from build123d import *

# Parameters (mm, degrees)
SKETCH2_W           = 18
SKETCH2_H           = 18
BOSS_EXTRUDE1_DEPTH = 18
SKETCH3_R           = 1.4224
CUT_EXTRUDE1_DEPTH  = 6.6
SKETCH4_R           = 1.4224
CUT_EXTRUDE2_DEPTH  = 6.6
SKETCH5_R           = 1.4224
CUT_EXTRUDE3_DEPTH  = 6.6
SKETCH6_W           = 16
SKETCH6_H           = 16
CUT_EXTRUDE4_DEPTH  = 16
SKETCH7_W           = 16
SKETCH7_H           = 16
CUT_EXTRUDE5_DEPTH  = 10


with BuildPart() as part:
    # Sketch2 → Boss-Extrude1 (new body)
    with BuildSketch(Plane(origin=(0, 0, 0), x_dir=(1, 0, 0), z_dir=(0, 1, 0))):
        Rectangle(SKETCH2_W, SKETCH2_H)
    extrude(amount=BOSS_EXTRUDE1_DEPTH)

    # Sketch3 → Cut-Extrude1 (cut)
    with BuildSketch(Plane(origin=(0, 18, 0), x_dir=(1, 0, 0), z_dir=(0, 1, 0))):
        Circle(SKETCH3_R)
    extrude(amount=-CUT_EXTRUDE1_DEPTH, mode=Mode.SUBTRACT)

    # Sketch4 → Cut-Extrude2 (cut)
    with BuildSketch(Plane(origin=(9, 0, 0), x_dir=(0, 0, -1), z_dir=(1, 0, 0))):
        with Locations((0, 9)):
            Circle(SKETCH4_R)
    extrude(amount=-CUT_EXTRUDE2_DEPTH, mode=Mode.SUBTRACT)

    # Sketch5 → Cut-Extrude3 (cut)
    with BuildSketch(Plane.XY.offset(9)):
        with Locations((0, 9)):
            Circle(SKETCH5_R)
    extrude(amount=-CUT_EXTRUDE3_DEPTH, mode=Mode.SUBTRACT)

    # Sketch6 → Cut-Extrude4 (cut)
    with BuildSketch(Plane(origin=(0, 0, -9), x_dir=(-1, 0, 0), z_dir=(0, 0, -1))):
        with Locations((1, 8)):
            Rectangle(SKETCH6_W, SKETCH6_H)
    extrude(amount=-CUT_EXTRUDE4_DEPTH, mode=Mode.SUBTRACT)

    # Sketch7 → Cut-Extrude5 (cut)
    with BuildSketch(Plane.ZY.offset(-7)):
        with Locations((-1, 8)):
            Rectangle(SKETCH7_W, SKETCH7_H)
    extrude(amount=-CUT_EXTRUDE5_DEPTH, mode=Mode.SUBTRACT)


solid = part.part
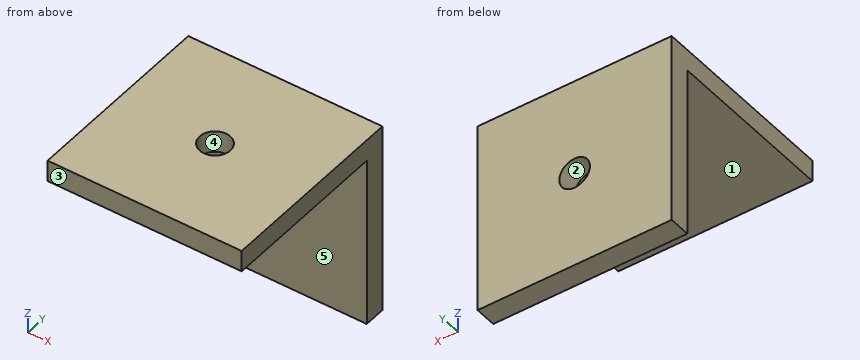
Model file for the job. Use its own axes, mm. Face numbers are marked on the shaded views. A direction names the side the tool comes from. Give positions to 0.01 mm unless a question says otherwise; leave off trailing zeros. Loops run counter-clockwise (first coordinate to the right, second up) from the corner with the lowest first, then second, coordinate; pieces in that order, holes last.
Item 1: Which spindle directions (+Z, -Z, +X, -X, +Y, -Y) get a long thin tool onto all of the face, cutting with end or side? Do the marked faces 4 and 5. Say none if no direction does.
Check values:
face 4: +Z, -Z
face 5: -Z, +X, -X, -Y
Item 2: Slice it at C-C (x = 0). Write the cut outline in (y, z).
Check values:
outline: (0, 7) - (7.58, 7) - (7.58, 9) - (0, 9) - close; (10.42, 7) - (16, 7) - (16, 1.42) - (18, 1.42) - (18, 9) - (10.42, 9) - close; (16, -9) - (18, -9) - (18, -1.42) - (16, -1.42) - close
Item 3: Drop flat-ended pins along their axis: P1, Ø5, axis at x = -2.5, y = 9, coming from the -Z side; P2, Ø2, axis at x = 4, z = 0.5, coming from the -Y side. Give the stop position or say it passes through.
Check values:
P1: stops at z = 7
P2: stops at y = 16
Item 4: Slice it at D-D (x = -3). Write the cut outline in (y, z), plus the area to 3 significant figures.
Check values:
outline: (0, 7) - (16, 7) - (16, -9) - (18, -9) - (18, 9) - (0, 9) - close
area: 68.0 mm2
Item 5: Slice it at B-B (y = 9). Write the cut outline in (x, z).
Check values:
outline: (-9, 7) - (-1.42, 7) - (-1.42, 9) - (-9, 9) - close; (1.42, 7) - (9, 7) - (9, 9) - (1.42, 9) - close
Item 6: Drill centre lines: line 1 along X through (y, z) = (17.55, 0); line 2 along Z through (x, y) = (-4.5, 5.5); line 3 along Y through (x, z) = (0, 7.6). Where is each one in solid material? Low to high.
Check values:
line 1: x = -9 to -1.42, 1.42 to 9
line 2: z = 7 to 9
line 3: y = 0 to 7.58, 10.42 to 18
Item 7: Mould opens along Z. For the marked faces 1, 2 and 3 say: +Z half, -Z half, draft (parallel to the pull), parting line (faces both ways), or undercut.
Check values:
face 1: -Z half
face 2: undercut
face 3: draft
Item 8: Slice it at A-A (z = 0). Write the cut outline in (x, y).
Check values:
outline: (-9, 16) - (-1.42, 16) - (-1.42, 18) - (-9, 18) - close; (1.42, 16) - (9, 16) - (9, 18) - (1.42, 18) - close
